Drawing for the job (mm, zero at the part's lowest x, y, z). A direction names the side the tool comes from. Give positions to 0.01 mm unless a question says otherwise; leave off trailing zeros. Order: outer loops, then holes, each group sorted by start corner. A loop starts at its lowest first (then second) coordinate and runs counter-clockwise, first axis right, second up. Notation, with made-up numbers: (-0.5, -38) - (32.5, -38) arc R22 cw to (32.5, -17) - close; hole circle Ø10 at (40, -1.5). An arc over 180 degrees is marked (long way). One line per item, written item: value.
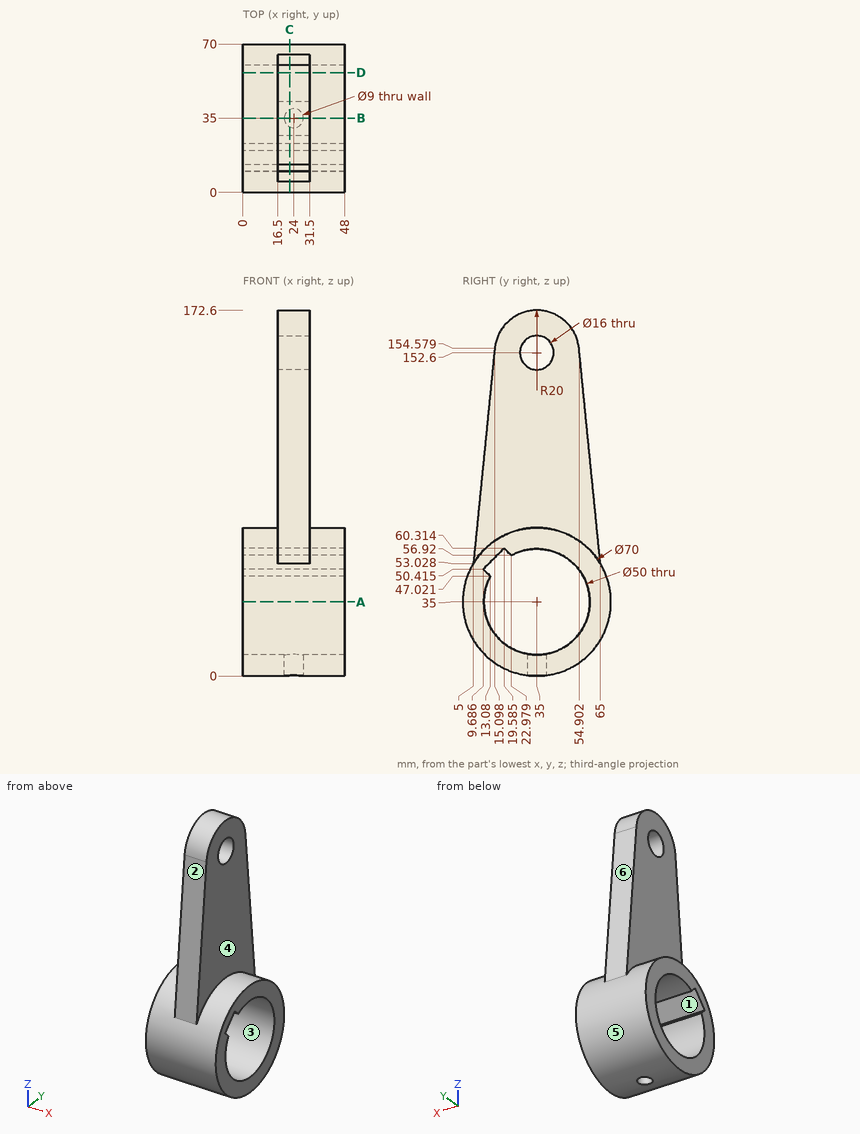
(1) 3-axis set-ups, long thin cutter, end or side, ignore diameter. For the marked faces 1 and 2: which of +Z, -Z, +X, -X, +Y, -Y reach the whole face in a straight line?
Completed:
face 1: +X, -X
face 2: +Z, +X, -X, -Y
(2) Slice it at B-B, the plane y = 35. Give the cut face in (x, z).
Completed:
outline: (0, 0) - (19.5, 0) - (19.5, 10) - (0, 10) - close; (0, 60) - (48, 60) - (48, 70) - (31.5, 70) - (31.5, 144.6) - (16.5, 144.6) - (16.5, 70) - (0, 70) - close; (16.5, 160.6) - (31.5, 160.6) - (31.5, 172.6) - (16.5, 172.6) - close; (28.5, 0) - (48, 0) - (48, 10) - (28.5, 10) - close
(3) Slice it at C-C, the plane x = 22. Give the cut face in (y, z) (1 decimal), and give its area (3 significant figures).
Completed:
outline: (5, 53) arc R35 ccw to (31, 0.2) - (31, 10.3) arc R25 cw to (13.1, 47) - (9.7, 50.4) - (19.6, 60.3) - (23, 56.9) arc R25 cw (long way) to (39, 10.3) - (39, 0.2) arc R35 ccw to (65, 53) - (54.9, 154.6) arc R20 ccw to (15.1, 154.6) - close; hole circle Ø16 at (35, 152.6)
area: 6,440 mm²
(4) Pull direction Y, two halves, no side cores. Call the marked faces 3, 4, 5 and 6: +Y half, -Y half, draft (parallel to the pull), parting line (faces both ways), or undercut.
Completed:
face 3: undercut
face 4: draft
face 5: parting line
face 6: +Y half
(5) Drill centre lines: line 1 (X direction, y = 14.5, z = 125); line 2 (Z direction, x = 26, y = 31.5) (1 decimal); line 3 (Z direction, x = 25, y = 49.5) (1 decimal). Where is each one in solid material? Low to high.
Completed:
line 1: 16.5 to 31.5
line 2: 59.8 to 145.4, 159.8 to 172.3
line 3: 3.1 to 14.6, 55.4 to 166.4
(6) Slice it at D-D, the plane y = 56.5. Give the cut face in (x, z).
Completed:
outline: (0, 7.38) - (48, 7.38) - (48, 22.24) - (0, 22.24) - close; (0, 47.76) - (48, 47.76) - (48, 62.62) - (31.5, 62.62) - (31.5, 138.51) - (16.5, 138.51) - (16.5, 62.62) - (0, 62.62) - close
(7) Pin check, flat tips, straight feed: P1, Ø8, axis at x = 28, z = 33, coming from the +Y side; P2, Ø10, axis at y = 62.5, z = 66, coming from the -X side; P3, Ø12, axis at x = 18, z = 142.5, coming from the -Y side. Stop position of each tip, or through.
Completed:
P1: y = 70
P2: x = 16.5
P3: y = 13.3
(8) Slice it at A-A, the plane z = 35. Give the cut face in (x, y), and give its area (3 significant figures).
Completed:
outline: (0, 0) - (48, 0) - (48, 10) - (0, 10) - close; (0, 60) - (48, 60) - (48, 70) - (0, 70) - close
area: 960 mm²
